Source: three-view drawing plus pictorial views. Frame: mm from the lowest corner of the part. A direction names the side the tool comes from. Round coordinates to 2 decimals unless told otherwise and drop trailing zeros. Loops run counter-clockwise (first coordinate to the right, second up) from the corner with the lowest first, then second, coordinate; pieces in that order, holes last. Notation, with made-up numbers: (-27, -13.5) -> (-1, -13.5) arc R21 cw to (-1, 23.5) -> close; hole circle Ø10 at (63.25, 77). An arc over 180 degrees is marked (long way). Answer in a Markdown table with one row per item. Add a question column.
Q1. Section D-D, the plane z = 72. Output: boundary loops of the cut face in (x, y), and give its area (3 significant figures).
Q2. Section C-C, the plane y = 95. Output: boundary loops of the cut face in (x, z), and give its area (3 significant figures).
Q3. Mould query, pull axis Z, two halves, no side actions, for the marked faces 1, 2 and 3. Classes: pulls with the +Z half, pulls with the -Z half, needs draft (parallel to the pull), parting line crosses it, or undercut.
Q4. Reachability of the marked faces 4, 5, 6, 7 and 8 from +Z, -Z, +X, -X, +Y, -Y: full face, straight path, thin tool, end or side. Return the list, or none.
Q5. Section B-B, the plane y = 69. Output: boundary loops of the cut face in (x, z).
Q6. Ray query, L1, parallel to Z at x = 22.5, y = 78.5; L2, parallel to X at y = 95, z = 61.5; L3, parallel to X at y = 58.5, z = 8.5. Return the intervals inside material, ascending. Write a range as from..to.
Q7. Section A-A, the plane x = 123. Output: boundary loops of the cut face in (y, z) (3 decimals).
Q8. Pin query (flat end, axial travel): pin 1 (12.5 mm diameter, centred on x = 115, y = 93, fed in from +Z); pin 2 (1.5 mm diameter, centred on x = 118.5, y = 46.5, fed in from +Z); pin 3 (25 mm diameter, centred on y = 80, z = 16, fed in from +X). Return the tip coordinate at first contact, or that it passes through.
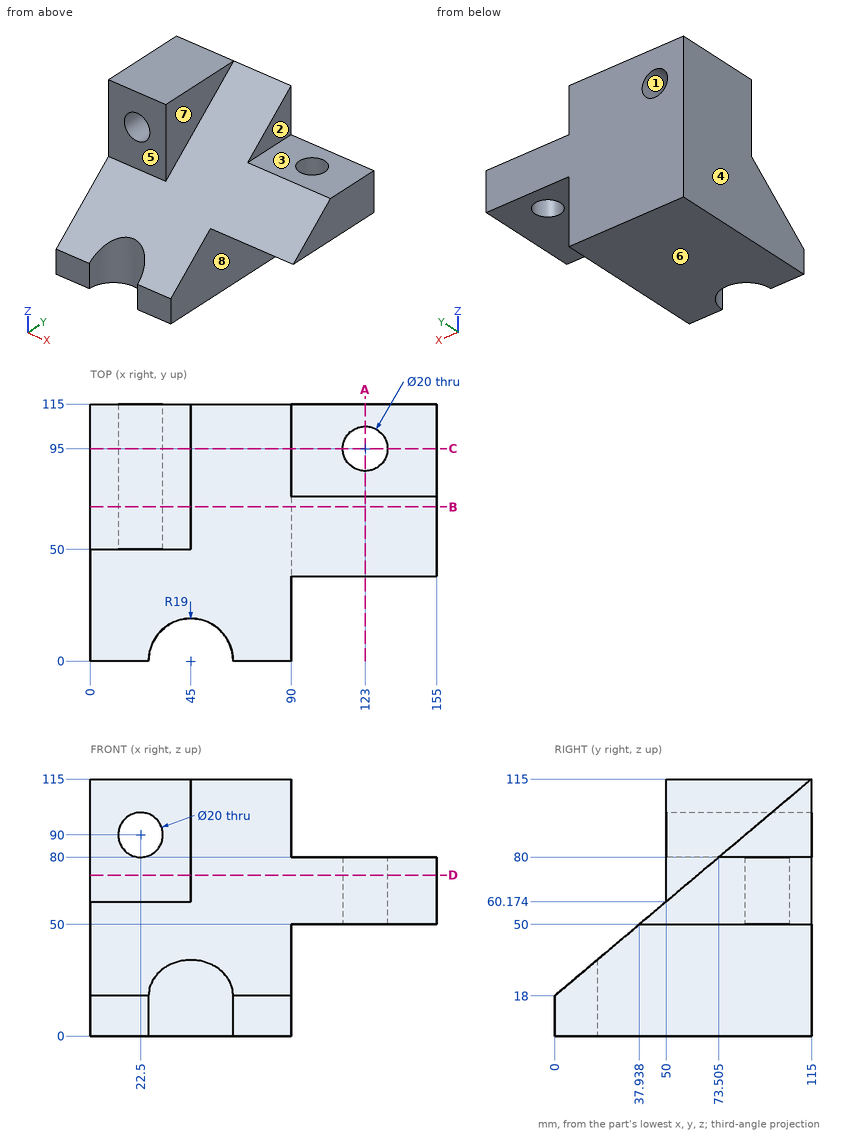
Answer block:
| question | item | result |
|---|---|---|
| 1 | outline | (0, 50) -> (45, 50) -> (45, 64.02) -> (155, 64.02) -> (155, 115) -> (0, 115) -> close; hole circle Ø20 at (123, 95) |
| 1 | area | 8,220 mm^2 |
| 2 | outline | (0, 0) -> (90, 0) -> (90, 50) -> (113, 50) -> (113, 80) -> (90, 80) -> (90, 98.13) -> (45, 98.13) -> (45, 115) -> (0, 115) -> close; (133, 50) -> (155, 50) -> (155, 80) -> (133, 80) -> close; hole circle Ø20 at (22.5, 90) |
| 2 | area | 10,600 mm^2 |
| 3 | face 1 | undercut |
| 3 | face 2 | needs draft |
| 3 | face 3 | pulls with the +Z half |
| 4 | face 4 | +Z, -Z, -X, +Y, -Y |
| 4 | face 5 | +Z, +X, -X, -Y |
| 4 | face 6 | -Z, +X, -X, +Y, -Y |
| 4 | face 7 | +Z, +X, -Y |
| 4 | face 8 | -Z, +X, +Y, -Y |
| 5 | outline | (0, 0) -> (90, 0) -> (90, 50) -> (155, 50) -> (155, 76.2) -> (45, 76.2) -> (45, 115) -> (0, 115) -> close; hole circle Ø20 at (22.5, 90) |
| 6 | L1 | 0..80, 100..115 |
| 6 | L2 | 0..113, 133..155 |
| 6 | L3 | 0..90 |
| 7 | outline | (37.938, 50) -> (85, 50) -> (85, 80) -> (73.505, 80) -> close; (105, 50) -> (115, 50) -> (115, 80) -> (105, 80) -> close |
| 8 | pin 1 | z = 80 |
| 8 | pin 2 | z = 57.85 |
| 8 | pin 3 | x = 90 |
